Here's how the part is built. I have some questions about the finished solid (model axes, mm). A direction names the side the tool comes from. Coordinates: 2 decimals unless noted, no trailing zeros. Loops run counter-clockwise (first coordinate to the right, second up) from the corner with the lowest first, then second, coordinate; pieces in that order, holes last. Notation, with made-up numbers: (12.5, 65) -> (48.5, 65) arc R21 cw to (48.5, 86) -> close; hole circle Ø5 at (-36.75, 7). An arc over 180 degrees is marked (long way). Answer as a JSON object with one key per item and string values. Group by question number.
1) I'm going to push flat-ended pins straight in: pin 1 (24.5 mm diameter, centred on x = 58.5, y = -188.5, fed in from +Z); pin 2 (10 mm diameter, centred on x = 177, z = 46.5, fed in from +Y); pin 3 (1 mm diameter, centred on x = 78.5, y = -166.5, fed in from -Z). Where does each tip first touch, or does it pass through?
2) I want a section at C-C (y = -117). Write out the boundary of the cut face in (x, z).
3) I want a section at A-A (x = 150). Write out the boundary of the cut face in (y, z).
4) Which directions (+Z, -Z, +X, -X, +Y, -Y) give clear straight access to the entire face, cutting with the end or side of a thin tool? Please do faces 1 (the flat face through (78, -42, 20)), 2 (the flat face through (203.846, -215, 85)), 3 (the cylindrical face through (125.024, -1.099, 169.86)), 4 (the flat face through (82, -79, 0)), 5 (the flat face through (-35, -128, 90)).
5) I want a section at D-D (y = -75). Write out the boundary of the cut face in (x, z), then the cut area to 3 significant figures.
6) I need wall thicknesses on probe 1 along X at (y, z) = (0, 175); probe 2 along Z at (x, y) = (155, -173); probe 3 along X at (y, z) = (-75, 172). Which ranges of each line are inside material? Lowest first, please. Write a range as [from, to].
7) If we mould it in two halves opening along X, with no side actions, what happens to faces 6 (the flat face through (77, -215, 183.462)), 7 (the cylindrical face through (16.844, -60.357, 169.86)), 8 (the cylindrical face through (-31, 37, 10))? For each: +X half, -X half, draft (parallel to the pull), parting line (faces both ways), or undercut.
Autodesk Inventor part; units mm, degrees
ref_plane "YZ Plane" through (0, 0, 0) normal (1, 0, 0) x (0, 1, 0)
ref_plane "XY Plane" through (0, 0, 0) normal (0, 0, 1) x (1, 0, 0)
sketch "Sketch1" plane through (0, 0, 0) normal (0, 0, 1) x (1, 0, 0)
  circle A0 centre (0, 0) radius 15
  circle A1 centre (150, 0) radius 25
  line L0 (-35, 45) -> (-35, -144.3782)
  circle A2 centre (43.934, -106.066) radius 15
  circle A3 centre (20.0962, -75) radius 15
  line L1 (195, 45) -> (-35, 45)
  line L2 (195, -205) -> (0, -205)
  line L3 (195, -205) -> (195, 45)
  line L4 (0, -205) -> (-35, -144.3782)
  line L5 (0, -205) -> (70, -205) construction
  dimension "d22" = 230
  dimension "d23" = 120
extrude "Extrusion1" add sketch "Sketch1" along normal blind 180
fillet "Fillet1" radius 50 1 edges at (-35, -144.3782, 90)
fillet "Fillet2" radius 20 1 edges at (-35, 45, 90)
fillet "Fillet3" radius 20 1 edges at (195, 45, 90)
fillet "Fillet4" radius 20 1 edges at (195, -205, 90)
fillet "Fillet5" radius 20 1 edges at (0, -205, 90)
sketch "Sketch2" plane through (-35, -130.9808, 0) normal (-1, 0, 0) x (0, 0, 1)
  line L0 (0, 155.9808) -> (180, 155.9808)
  line L1 (0, 155.9808) -> (0, 0)
  line L2 (180, 155.9808) -> (180, 0)
  line L3 (0, 175) -> (0, -75)
  line L4 (0, -75) -> (20, -75)
  line L5 (20, -75) -> (20, -25)
  line L6 (20, -25) -> (160, -25)
  line L7 (160, -25) -> (160, -75)
  line L8 (160, -75) -> (180, -75)
  line L9 (180, -75) -> (180, 175)
  line L10 (180, 175) -> (160, 175)
  line L11 (160, 175) -> (160, 5)
  line L12 (160, 5) -> (20, 5)
  line L13 (20, 5) -> (20, 175)
  line L14 (20, 175) -> (0, 175)
  point P0 (0, 130.9808)
  dimension "d31" = 250
  dimension "d32" = 20
  dimension "d33" = 50
  dimension "d34" = 140
  dimension "d35" = 170
extrude "Extrusion2" cut sketch "Sketch2" against normal blind 230 contours L3 L14 L13 L0 | L0 L13 L12 L11 L2 L9 L8 L7 L6 L5 L4 L3 L1 | L11 L10 L9 L0 keep common part
sketch "Sketch3" plane through (0, 0, 180) normal (0, 0, 1) x (1, 0, 0)
  circle A0 centre (43.934, -106.066) radius 15
  circle A1 centre (43.934, -106.066) radius 15
extrude "Extrusion3" add sketch "Sketch3" against normal blind 20
sketch "Sketch4" plane through (0, 0, 0) normal (0, 0, -1) x (-1, 0, 0)
  circle A0 centre (-43.934, -106.066) radius 15
  circle A1 centre (-43.934, -106.066) radius 15
extrude "Extrusion4" add sketch "Sketch4" against normal blind 20
ref_plane "Work Plane1" through (175, -205, 20) normal (0, 1, 0) x (-1, 0, 0)
sketch "Sketch6" plane through (175, -205, 20) normal (0, 1, 0) x (-1, 0, 0)
  line L0 (-19.2308, -36.5385) -> (221.1538, -36.5385)
  line L1 (221.1538, -36.5385) -> (221.1538, 163.4615)
  line L2 (221.1538, 163.4615) -> (-28.8462, 163.4615)
  line L3 (-28.8462, 163.4615) -> (-28.8462, -36.5385)
  line L4 (-28.8462, -36.5385) -> (-19.2308, -36.5385)
  point P0 (175, -20)
  dimension "d55" = 250
  dimension "d56" = 200
extrude "Extrusion6" add sketch "Sketch6" against normal blind 20
sketch "Sketch7" plane through (175, -225, 20) normal (0, -1, 0) x (1, 0, 0)
  line L0 (-221.1538, -36.5385) -> (28.8462, -36.5385)
  line L1 (28.8462, -36.5385) -> (28.8462, 163.4615)
  line L2 (28.8462, 163.4615) -> (-221.1538, 163.4615)
  line L3 (-221.1538, 163.4615) -> (-221.1538, -36.5385)
  point P0 (-175, -20)
properties part number "sketss"
Determined:
{
 "1": {"pin 1": "z = 180", "pin 2": "y = -125.98", "pin 3": "z = 0"},
 "2": {"outline": "(-35, 0) -> (195, 0) -> (195, 20) -> (-35, 20) -> close; (-35, 160) -> (195, 160) -> (195, 180) -> (-35, 180) -> close"},
 "3": {"outline": "(-225, -16.54) -> (-205, -16.54) -> (-205, 0) -> (-25, 0) -> (-25, 20) -> (-125.98, 20) -> (-125.98, 160) -> (-25, 160) -> (-25, 180) -> (-205, 180) -> (-205, 183.46) -> (-225, 183.46) -> close; (25, 0) -> (44.02, 0) -> (44.02, 20) -> (25, 20) -> close; (25, 160) -> (44.02, 160) -> (44.02, 180) -> (25, 180) -> close; hole (-205, 20) -> (-155.98, 20) -> (-155.98, 160) -> (-205, 160) -> close"},
 "4": {"face 1": "+X, -X, +Y", "face 2": "+Z, -Z, +X, +Y, -Y", "face 3": "+Z, -Z", "face 4": "-Z, +X, -X, +Y", "face 5": "+Z, -Z, -X, +Y"},
 "5": {"outline": "(-35, 0) -> (5.1, 0) -> (5.1, 20) -> (-35, 20) -> close; (-35, 160) -> (5.1, 160) -> (5.1, 180) -> (-35, 180) -> close; (35.1, 0) -> (195, 0) -> (195, 20) -> (35.1, 20) -> close; (35.1, 160) -> (195, 160) -> (195, 180) -> (35.1, 180) -> close", "area": "8,000 mm^2"},
 "6": {"probe 1": "[-35, -15], [15, 125], [175, 195]", "probe 2": "[0, 20], [160, 180]", "probe 3": "[-35, 5.1], [35.1, 195]"},
 "7": {"face 6": "draft", "face 7": "undercut", "face 8": "-X half"}
}
